Check sheet for the modelled part. Datum: model origin and axes. Units: mm. A direction names the side the tool comes from. Round coordinates to 2 decimals unless told otherwise and drop trailing zeros. Loops run counter-clockwise (first coordinate to the right, second up) from the corner with the lowest first, then second, coordinate; pieces in that order, holes last. Notation, with made-up numbers: (32.5, -9) - (63.5, -9) arc R35 cw to (63.5, 28) - close; hole circle Ø7 at (49, 25). An arc over 180 degrees is marked (long way). Return JSON: item names as keys, results as strings.
from build123d import *

# Parameters (mm, degrees)
SKETCH1_W           = 30
SKETCH1_H           = 7
BOSS_EXTRUDE1_DEPTH = 20
SKETCH2_R           = 1.5
CUT_EXTRUDE1_DEPTH  = 2
SKETCH3_R           = 1.5
CUT_EXTRUDE2_DEPTH  = 2


with BuildPart() as part:
    # Sketch1 → Boss-Extrude1 (new body)
    with BuildSketch(Plane.XY):
        with Locations((15, 3.5)):
            Rectangle(SKETCH1_W, SKETCH1_H)
    extrude(amount=BOSS_EXTRUDE1_DEPTH)

    # Sketch2 → Cut-Extrude1 (cut)
    with BuildSketch(Plane.XY.offset(20)):
        with Locations((15, 3.5)):
            Circle(SKETCH2_R)
    extrude(amount=-CUT_EXTRUDE1_DEPTH, mode=Mode.SUBTRACT)

    # Sketch3 → Cut-Extrude2 (cut)
    with BuildSketch(Plane(origin=(0, 7, 0), x_dir=(1, 0, 0), z_dir=(0, 1, 0))):
        with Locations((7.5, -10)):
            Circle(SKETCH3_R)
        with Locations((22.5, -10)):
            Circle(SKETCH3_R)
    extrude(amount=-CUT_EXTRUDE2_DEPTH, mode=Mode.SUBTRACT)


solid = part.part
Q1. Sectioned sample at A-A (y = 5.75). Enter the section's corners in (x, z), plus the area to 3 significant figures.
Answer key:
{"outline": "(0, 0) - (30, 0) - (30, 20) - (0, 20) - close; hole circle Ø3 at (7.5, 10); hole circle Ø3 at (22.5, 10)", "area": "586 mm²"}
Q2. Draft check along X on faces 1 (the face through (15, 0, 10)), 2 (the face through (13.5, 3.57, 19.01)), 3 (the face through (30, 3, 10)), 4 (the face through (6.3, 6, 10.9)). Enter one of: released by +X, released by -X, zero draft, split by the parting line, or undercut.
Answer key:
{"face 1": "zero draft", "face 2": "undercut", "face 3": "released by +X", "face 4": "undercut"}
Q3. Tool access check on faces 5 (the face through (7, 5, 10)), 6 (the face through (15, 7, 10)), 7 (the face through (15, 4, 18)). Record the directions out of +Z, -Z, +X, -X, +Y, -Y that give a thin tool (end or side, any length) a straight path to the whole face; none if there is none.
Answer key:
{"face 5": "+Y", "face 6": "+Z, -Z, +X, -X, +Y", "face 7": "+Z"}
Q4. Sectioned sample at D-D (x = 8.25). Enter the section's corners in (y, z).
Answer key:
{"outline": "(0, 0) - (7, 0) - (7, 8.7) - (5, 8.7) - (5, 11.3) - (7, 11.3) - (7, 20) - (0, 20) - close"}
Q5. Scan lines: probe 1 along X at (y, z) = (5.8, 10); probe 2 along Z at (x, y) = (7.5, 5.5); probe 3 along Y at (x, z) = (15, 18.5). Record each from-to range of solid material in increasing order. Write a range as [from, to].
Answer key:
{"probe 1": "x = [0, 6], [9, 21], [24, 30]", "probe 2": "z = [0, 8.5], [11.5, 20]", "probe 3": "y = [0, 2], [5, 7]"}
Q6. Sectioned sample at B-B (z = 10). Enter the section's corners in (x, y).
Answer key:
{"outline": "(0, 0) - (30, 0) - (30, 7) - (24, 7) - (24, 5) - (21, 5) - (21, 7) - (9, 7) - (9, 5) - (6, 5) - (6, 7) - (0, 7) - close"}
Q7. Sectioned sample at C-C (x = 22.5). Enter the section's corners in (y, z), plus the area to 3 significant figures.
Answer key:
{"outline": "(0, 0) - (7, 0) - (7, 8.5) - (5, 8.5) - (5, 11.5) - (7, 11.5) - (7, 20) - (0, 20) - close", "area": "134 mm²"}
Q8. Depth check by flat-ended pin: P1, Ø1.5, axis at x = 22, z = 9.5, coming from the +Y side. Enter the tip coordinate at first touch or a pass-through.
Answer key:
{"P1": "stops at y = 5"}
